Source: CAD feature listing. Evaluate the final solid. Frame: model axes, mm. Face numbers are marked on the shaded views. Give positions to 0.01 mm unless a question says otherwise; leave off trailing zeros. Order: outer loops, then holes, each group sorted by start corner. A loop starts at its lowest first (then second) coordinate and runs counter-clockwise, first axis right, second up. Notation, with made-up numbers: (84, 28) -> (96, 28) arc R32 cw to (96, 60) -> close; hole circle Ø1 at (-10, 43.5). An arc over 180 degrees is marked (long way). Answer in a Markdown table with one row per item.
```python
from build123d import *

# Parameters (mm, degrees)
SKETCH1_R           = 42
BOSS_EXTRUDE1_DEPTH = 80
SKETCH7_R           = 42
BOSS_EXTRUDE2_DEPTH = 19
SKETCH8_R           = 40.2
BATTERY_SLOT_DEPTH  = 19
SKETCH10_W          = 80.3
SKETCH10_H          = 67
CUT_EXTRUDE6_DEPTH  = 19
SKETCH11_R          = 42
BOSS_EXTRUDE3_DEPTH = 20
SKETCH12_R          = 42
BOSS_EXTRUDE4_DEPTH = 50
SKETCH13_R          = 40.2
CUT_EXTRUDE7_DEPTH  = 50
SKETCH14_R          = 42
BOSS_EXTRUDE5_DEPTH = 35
SKETCH15_R          = 40.2
RPI_SLOT_DEPTH      = 25
SKETCH16_W          = 68
SKETCH16_H          = 64
CUT_EXTRUDE9_DEPTH  = 25
SKETCH17_R          = 42
BOSS_EXTRUDE6_DEPTH = 20
SKETCH18_R          = 42
BOSS_EXTRUDE7_DEPTH = 175


with BuildPart() as part:
    # Sketch1 → Boss-Extrude1 (new body)
    with BuildSketch(Plane(origin=(0, 0, 0), x_dir=(1, 0, 0), z_dir=(0, 1, 0))):
        with Locations(Location((0, 0, 0), (0, 0, 270))):
            Circle(SKETCH1_R)
    extrude(amount=BOSS_EXTRUDE1_DEPTH)

    # Sketch7 → Boss-Extrude2 (add)
    with BuildSketch(Plane(origin=(0, 80, 0), x_dir=(1, 0, 0), z_dir=(0, 1, 0))):
        with Locations(Location((0, 0, 0), (0, 0, 270))):
            Circle(SKETCH7_R)
    extrude(amount=BOSS_EXTRUDE2_DEPTH)

    # Sketch8 → Battery slot (cut)
    with BuildSketch(Plane(origin=(0, 99, 0), x_dir=(1, 0, 0), z_dir=(0, 1, 0))):
        with Locations(Location((0, 0, 0), (0, 0, 270))):
            Circle(SKETCH8_R)
    extrude(amount=-BATTERY_SLOT_DEPTH, mode=Mode.SUBTRACT)

    # Sketch10 → Cut-Extrude6 (cut)
    with BuildSketch(Plane(origin=(0, 99, 0), x_dir=(1, 0, 0), z_dir=(0, 1, 0))):
        with Locations((0, -31.495629775)):
            Rectangle(SKETCH10_W, SKETCH10_H)
    extrude(amount=-CUT_EXTRUDE6_DEPTH, mode=Mode.SUBTRACT)

    # Sketch11 → Boss-Extrude3 (add)
    with BuildSketch(Plane(origin=(0, 99, 0), x_dir=(1, 0, 0), z_dir=(0, 1, 0))):
        with Locations(Location((0, 0, 0), (0, 0, 270))):
            Circle(SKETCH11_R)
    extrude(amount=BOSS_EXTRUDE3_DEPTH)

    # Sketch12 → Boss-Extrude4 (add)
    with BuildSketch(Plane(origin=(0, 119, 0), x_dir=(1, 0, 0), z_dir=(0, 1, 0))):
        with Locations(Location((0, 0, 0), (0, 0, 270))):
            Circle(SKETCH12_R)
    extrude(amount=BOSS_EXTRUDE4_DEPTH)

    # Sketch13 → Cut-Extrude7 (cut)
    with BuildSketch(Plane(origin=(0, 169, 0), x_dir=(1, 0, 0), z_dir=(0, 1, 0))):
        with Locations(Location((0, 0, 0), (0, 0, 270))):
            Circle(SKETCH13_R)
    extrude(amount=-CUT_EXTRUDE7_DEPTH, mode=Mode.SUBTRACT)

    # Sketch14 → Boss-Extrude5 (add)
    with BuildSketch(Plane(origin=(0, 169, 0), x_dir=(1, 0, 0), z_dir=(0, 1, 0))):
        with Locations(Location((0, 0, 0), (0, 0, 270))):
            Circle(SKETCH14_R)
    extrude(amount=BOSS_EXTRUDE5_DEPTH)

    # Sketch15 → RPI Slot (cut)
    with BuildSketch(Plane(origin=(0, 204, 0), x_dir=(1, 0, 0), z_dir=(0, 1, 0))):
        with Locations(Location((0, 0, 0), (0, 0, 270))):
            Circle(SKETCH15_R)
    extrude(amount=-RPI_SLOT_DEPTH, mode=Mode.SUBTRACT)

    # Sketch16 → Cut-Extrude9 (cut)
    with BuildSketch(Plane(origin=(0, 204, 0), x_dir=(1, 0, 0), z_dir=(0, 1, 0))):
        with Locations((0, 18)):
            Rectangle(SKETCH16_W, SKETCH16_H)
    extrude(amount=-CUT_EXTRUDE9_DEPTH, mode=Mode.SUBTRACT)

    # Sketch17 → Boss-Extrude6 (add)
    with BuildSketch(Plane(origin=(0, 204, 0), x_dir=(1, 0, 0), z_dir=(0, 1, 0))):
        with Locations(Location((0, 0, 0), (0, 0, 270))):
            Circle(SKETCH17_R)
    extrude(amount=BOSS_EXTRUDE6_DEPTH)

    # Sketch18 → Boss-Extrude7 (add)
    with BuildSketch(Plane(origin=(0, 224, 0), x_dir=(1, 0, 0), z_dir=(0, 1, 0))):
        with Locations(Location((0, 0, 0), (0, 0, 270))):
            Circle(SKETCH18_R)
    extrude(amount=BOSS_EXTRUDE7_DEPTH)


solid = part.part
```
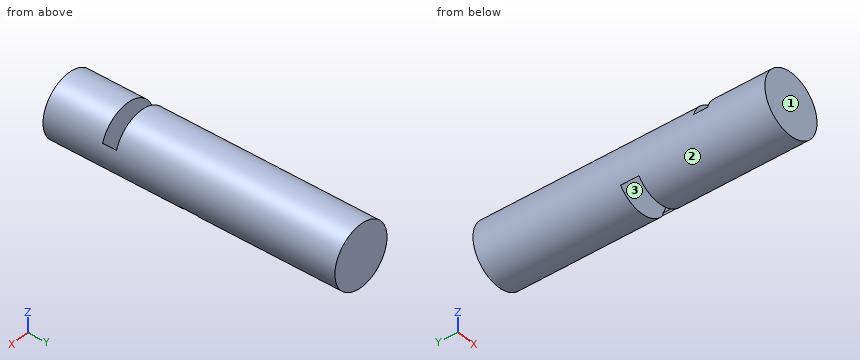
(1) Section query B-B (x = 0). Return the cut outline in (y, z), plus the area to 3 significant figures.
A:
| item | result |
|---|---|
| outline | (0, -42) -> (179, -42) -> (179, 40.2) -> (204, 40.2) -> (204, -42) -> (399, -42) -> (399, 42) -> (99, 42) -> (99, -40.2) -> (80, -40.2) -> (80, 42) -> (0, 42) -> close; hole (119, -40.2) -> (169, -40.2) -> (169, 40.2) -> (119, 40.2) -> close |
| area | 25,900 mm^2 |
(2) Section query D-D (y = 215). Return the cut outline in (x, z), plus the area to 3 significant figures.
A:
| item | result |
|---|---|
| outline | circle Ø84 at (0, 0) |
| area | 5,540 mm^2 |
(3) Pull-direction query (X, two-part tool) for the marked faces 1, 2 and 3; classes: +X half, -X half, draft (parallel to the pull), parting line (faces both ways), or undercut.
A:
| item | result |
|---|---|
| face 1 | draft |
| face 2 | parting line |
| face 3 | undercut |
(4) First-contact query: pin 1 Ø2 at (y, z) = (174, -1) entering from +X; pin 2 Ø10 at (x, y) = (32.5, 74.5) entering from +Z; pin 3 Ø1.5 at (x, y) = (-4.5, 58.5) entering from -Z. Flat tips, straight axial feed; report the tip coordinate or a pass-through.
A:
| item | result |
|---|---|
| pin 1 | stops at x = 42 |
| pin 2 | stops at z = 31.75 |
| pin 3 | stops at z = -41.83 |
(5) Section query A-A (z = 35.5). Return the cut outline in (x, y).
A:
| item | result |
|---|---|
| outline | (-22.44, 0) -> (22.44, 0) -> (22.44, 80) -> (-22.44, 80) -> close; (-22.44, 99) -> (22.44, 99) -> (22.44, 399) -> (-22.44, 399) -> close; hole (-18.86, 119) -> (18.86, 119) -> (18.86, 169) -> (-18.86, 169) -> close; hole (-18.86, 179) -> (18.86, 179) -> (18.86, 204) -> (-18.86, 204) -> close |
(6) Ray query, probe 1 along Y at (x, z) = (-11, -27); probe 2 along X at (y, z) = (134, 0); probe 3 along Z at (x, y) = (-0.5, 65.5). Return the intervals inside material, ascending.
A:
| item | result |
|---|---|
| probe 1 | y = 0 to 80, 99 to 119, 169 to 179, 204 to 399 |
| probe 2 | x = -42 to -40.2, 40.2 to 42 |
| probe 3 | z = -42 to 42 |
(7) Section query C-C (z = -1.5). Return the cut outline in (x, y), plus the area to 3 significant figures.
A:
| item | result |
|---|---|
| outline | (-41.97, 0) -> (41.97, 0) -> (41.97, 399) -> (-41.97, 399) -> close; hole (-40.17, 80) -> (40.17, 80) -> (40.17, 99) -> (-40.17, 99) -> close; hole (-40.17, 119) -> (40.17, 119) -> (40.17, 169) -> (-40.17, 169) -> close; hole (-40.17, 179) -> (40.17, 179) -> (40.17, 204) -> (-40.17, 204) -> close |
| area | 25,900 mm^2 |
